Could you check a few things on this model? Use its own coordinates, in mm. Give positions to 0.01 mm unless a question says otherwise; leave off trailing zeros. Order: outer loops, then holes, each group sorted by start corner. A loop starts at its lowest first (then second) coordinate and runs counter-clockwise, first axis right, second up.
from build123d import *

# Parameters (mm, degrees)
PAD008_DEPTH               = 22
POCKET008_DEPTH            = 4
BODY004023_PLACEMENT_ANGLE = 90


with BuildPart() as part:
    # Sketch014 → Pad008 (new body)
    with BuildSketch(Plane.XY):
        Polygon((9.2084513411, 14.8813448283), (10.0276033854, 15.4549212646), (18.6312499306, 3.1676406003), (17.8120978864, 2.594064164), align=None)
    pad008 = extrude(amount=-PAD008_DEPTH)

    # Mirrored: Pad008 across face of Pad008
    add(pad008.mirror(Plane(origin=(13.9198506359, 9.0244927143, -22), x_dir=(1, 0, 0), z_dir=(0, 0, -1))))

    # Sketch027 → Pocket008 (cut)
    with BuildSketch(Plane.XY):
        Polygon((9.2084513411, 14.8813448283), (10.0276033854, 15.4549212646), (12.0351209126, 12.5878891096), (11.2159688683, 12.0143126733), align=None)
        Polygon((18.6312499306, 3.1676406003), (17.8120978864, 2.594064164), (15.8045803591, 5.461096319), (16.6237324034, 6.0346727553), align=None)
    pocket008 = extrude(amount=-POCKET008_DEPTH, mode=Mode.SUBTRACT)

    # Mirrored001: Pocket008 across face of Pad008
    add(pocket008.mirror(Plane(origin=(13.9198506359, 9.0244927143, -22), x_dir=(1, 0, 0), z_dir=(0, 0, -1))), mode=Mode.SUBTRACT)


with BuildPart() as part_1:
    # Body004023 placement: moved
    add(part.part.rotate(Axis((0, 0, 0), (0, 0, 1)), BODY004023_PLACEMENT_ANGLE))


solid = part_1.part
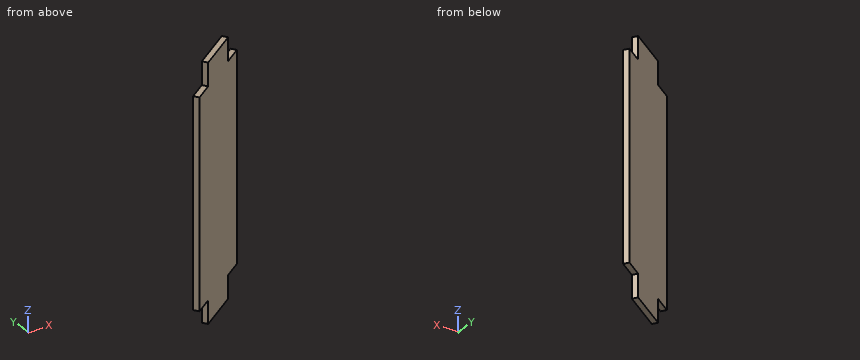
Item 1: Imagine slicing it at B-B on x = -13.5. List the corners of the cut face in (y, z) for me, then the cut area to 3 significant figures.
Findings:
outline: (10.18, -40) - (11.4, -40) - (11.4, -4) - (10.18, -4) - close
area: 43.9 mm2
Item 2: For pin 1 (5 mm diameter, centred on x = -10.5, z = -20.5, fed in from +Y); pin 2 (1 mm diameter, centred on x = -7, z = -16.5, fed in from -Y); pin 3 (5 mm diameter, centred on y = 11.5, z = -21, fed in from -X), each with a flat end and sliding along its axis, tell me the tip position at first contact or that it passes through.
Findings:
pin 1: stops at y = 15.25
pin 2: stops at y = 14.38
pin 3: stops at x = -15.45
Item 3: Imagine slicing it at A-A on z = -25. List the corners of the cut face in (x, y) for me, then the cut area to 3 significant figures.
Findings:
outline: (-15.45, 10.03) - (-14.88, 9.21) - (-2.59, 17.81) - (-3.17, 18.63) - close
area: 15.0 mm2
Item 4: Please list where these lines run through material, in increasing order: line 1 along Y through (x, z) = (-7.5, -25); line 2 along X through (y, z) = (18.25, -11); line 3 along X through (y, z) = (11.5, -23).
Findings:
line 1: y = 14.38 to 15.6
line 2: x = -3.71 to -2.9
line 3: x = -13.35 to -11.61
